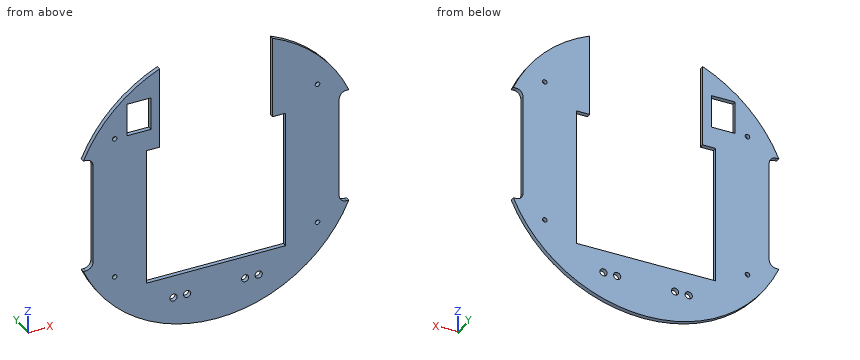
from build123d import *

# Parameters (mm, degrees)
SKETCH_1_W      = 16.4
SKETCH_1_H      = 22.8
SKETCH_1_R      = 1.6
SKETCH_1_R_2    = 2.5
EXTRUDE_1_DEPTH = 3


with BuildPart() as part:
    # 草圖1 → 填料-伸長1 (new body)
    with BuildSketch(Plane(origin=(0, 0, 0), x_dir=(1, 0, 0), z_dir=(0, 1, 0))):
        with BuildLine():
            ThreePointArc((39, -92.081485653), (70.324780895, -71.094480742), (91.651513899, -40))
            Line((91.651513899, -40), (90, -40))
            ThreePointArc((90, -40), (86.464466094, -38.535533906), (85, -35))
            Line((85, -35), (85, 35))
            ThreePointArc((85, 35), (86.464466094, 38.535533906), (90, 40))
            Line((90, 40), (91.651513899, 40))
            ThreePointArc((91.651513899, 40), (0, 100), (-91.651513899, 40))
            Line((-91.651513899, 40), (-90, 40))
            ThreePointArc((-90, 40), (-86.464466094, 38.535533906), (-85, 35))
            Line((-85, 35), (-85, -35))
            ThreePointArc((-85, -35), (-86.464466094, -38.535533906), (-90, -40))
            Line((-90, -40), (-91.651513899, -40))
            ThreePointArc((-91.651513899, -40), (-70.324780895, -71.094480742), (-39, -92.081485653))
            Line((-39, -92.081485653), (-39, -35.26))
            Line((-39, -35.26), (-48, -35.26))
            Line((-48, -35.26), (-48, 60.74))
            Line((-48, 60.74), (48, 60.74))
            Line((48, 60.74), (48, -35.26))
            Line((48, -35.26), (39, -35.26))
            Line((39, -35.26), (39, -92.081485653))
        make_face()
        with Locations((-53.204834595, -61.300870246)):
            Rectangle(SKETCH_1_W, SKETCH_1_H, mode=Mode.SUBTRACT)
        with Locations(Location((-70, -50, 0), (0, 0, 270))):
            Circle(SKETCH_1_R, mode=Mode.SUBTRACT)
        with Locations(Location((70, -50, 0), (0, 0, 270))):
            Circle(SKETCH_1_R, mode=Mode.SUBTRACT)
        with Locations(Location((-70, 50, 0), (0, 0, 270))):
            Circle(SKETCH_1_R, mode=Mode.SUBTRACT)
        with Locations(Location((-29.4, 76.443273383, 0), (0, 0, 270))):
            Circle(SKETCH_1_R_2, mode=Mode.SUBTRACT)
        with Locations(Location((-20, 76.443273383, 0), (0, 0, 270))):
            Circle(SKETCH_1_R_2, mode=Mode.SUBTRACT)
        with Locations(Location((20, 76.443273383, 0), (0, 0, 270))):
            Circle(SKETCH_1_R_2, mode=Mode.SUBTRACT)
        with Locations(Location((29.4, 76.443273383, 0), (0, 0, 270))):
            Circle(SKETCH_1_R_2, mode=Mode.SUBTRACT)
        with Locations(Location((70, 50, 0), (0, 0, 270))):
            Circle(SKETCH_1_R, mode=Mode.SUBTRACT)
    extrude(amount=EXTRUDE_1_DEPTH)


solid = part.part
Build history of the part. All positions in model axes, mm. Round coordinates to 2 decimals unless told otherwise and drop trailing zeros. Write each loop counter-clockwise with the first axis right and the second up, starting at its lowest first coordinate (ties: lowest second). Pieces come first, ordered by that corner, then holes. Notation, with made-up numbers: M 27.5,-12 L 55.5,-12 A18 cw 55.5,6 Z; hole C -16,1 d8. An arc over 180 degrees is marked long. Answer as a JSON object with one key per item and string values. Group by question number.
(1) Cut at B-B (y = 1.55). Give the number of separate pieces and of enclosed holes in the cut face, and give its area (3 significant figures).
(2) Drill centre lines: L1, parallel to Z at x = -70, y = 1.2; L2, parallel to X at y = 0.65, z = -50; L3, parallel to X at y = 1.15, z = -77.5. Where is each one in solid material? Low to high.
(3) Cut at C-C (x = -29.4). Give the cut face in (y, z).
(4) Cut at A-A (z = 16). Give the cut face in (x, y), and give its area (3 significant figures).
(5) Cut at D-D (x = -65). Give the cut face in (y, z).
(6) Flat gauge pins, fed straight in: pin 1 (1.9 mm diameter, centred on x = -70, z = -50, fed in from -Y); pin 2 (1 mm diameter, centred on x = 55, y = 0.5, fed in from +Z); pin 3 (1.5 mm diameter, centred on y = 1.5, z = 64.5, fed in from -X); pin 4 (0.9 mm diameter, centred on x = 45.5, y = 1.5, fed in from -Z). Where does each tip first touch, or does it go through?
Responses:
{
 "1": {"separate pieces": "1", "enclosed holes": "9", "area": "14,900 mm2"},
 "2": {"L1": "z = -71.41 to -51.6, -48.4 to 48.4, 51.6 to 71.41", "L2": "x = -86.6 to -71.6, -68.4 to -48, 48 to 68.4, 71.6 to 86.6", "L3": "x = -63.2 to -31.67, -27.13 to -22.27, -17.73 to 17.73, 22.27 to 27.13, 31.67 to 63.2"},
 "3": {"outline": "M 0,-95.58 L 3,-95.58 L 3,-78.94 L 0,-78.94 Z; M 0,-73.94 L 3,-73.94 L 3,-60.74 L 0,-60.74 Z"},
 "4": {"outline": "M -85,0 L -48,0 L -48,3 L -85,3 Z; M 48,0 L 85,0 L 85,3 L 48,3 Z", "area": "222 mm2"},
 "5": {"outline": "M 0,-75.99 L 3,-75.99 L 3,75.99 L 0,75.99 Z"},
 "6": {"pin 1": "passes through", "pin 2": "stops at z = 83.84", "pin 3": "stops at x = -77.05", "pin 4": "stops at z = -89.28"}
}
